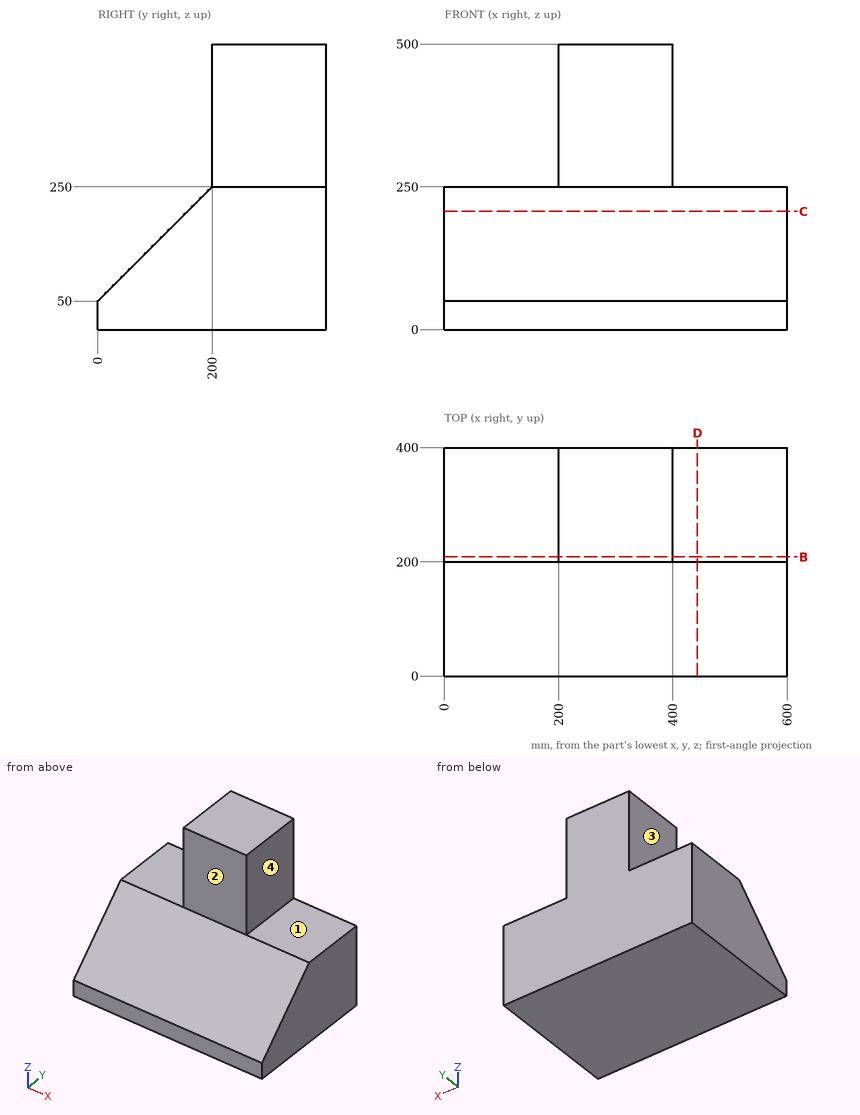
Part print with two shaded views. Sizes in mm from the minimum x, y, z corner. A direction names the side the tool comes from. Round coordinates to 2 decimals unless told otherwise and drop trailing zeros. Write each loop counter-clockwise with the first axis right and the second up, starting at its lowest first coordinate (ties: lowest second). Pieces come first, ordered by that corner, then holes. Notation, with made-up numbers: (-34.5, -24.5) - (-27.5, -24.5) arc R15 cw to (-27.5, -7.5) - close; hole circle Ø8 at (84, -9). An arc over 180 degrees is marked (long way). Answer as CSV lines item,"result".
Q1. Tool access for the marked faces 1, 2, 3 and 4: list every direction of +Z, -Z, +X, -X, +Y, -Y with a clear straight run to the whole face (end or side of a thin tool).
Report:
face 1,"+Z, +X, +Y, -Y"
face 2,"+Z, +X, -X, -Y"
face 3,"+Z, -X, +Y, -Y"
face 4,"+Z, +X, +Y, -Y"
Q2. Cut at C-C (z = 207). Write the cut outline in (x, y), and give its area (3 significant figures).
Report:
outline,"(0, 157) - (600, 157) - (600, 400) - (0, 400) - close"
area,"146,000 mm^2"
Q3. Cut at D-D (x = 443). Write the cut outline in (y, z).
Report:
outline,"(0, 0) - (400, 0) - (400, 250) - (200, 250) - (0, 50) - close"
Q4. Drop flat-ended pins along their axis: pin 1 (4 mm diameter, centred on y = 312, z = 283, fed in from -X); pin 2 (2 mm diameter, centred on x = 328.5, z = 301.5, fed in from -Y). Give the stop position or say it passes through.
Report:
pin 1,"stops at x = 200"
pin 2,"stops at y = 200"
Q5. Cut at B-B (y = 208.5). Write the cut outline in (x, z).
Report:
outline,"(0, 0) - (600, 0) - (600, 250) - (400, 250) - (400, 500) - (200, 500) - (200, 250) - (0, 250) - close"
Q6. Drill centre lines: probe 1 along Y at (x, z) = (203.5, 463); probe 2 along Z at (x, y) = (159, 322). Where is each one in solid material? Low to high. Write a range as [from, to].
Report:
probe 1,"y = [200, 400]"
probe 2,"z = [0, 250]"
